Input: dimensioned drawing with shaded views. Units: mm. Origin: part minimum x, y, z. Give positions to 0.01 mm unless a question says otherwise; leave off trailing zeros. Loops run counter-clockwise (first coordinate to the right, second up) from the corner with the lowest first, then second, coordinate; pieces in that order, holes last.
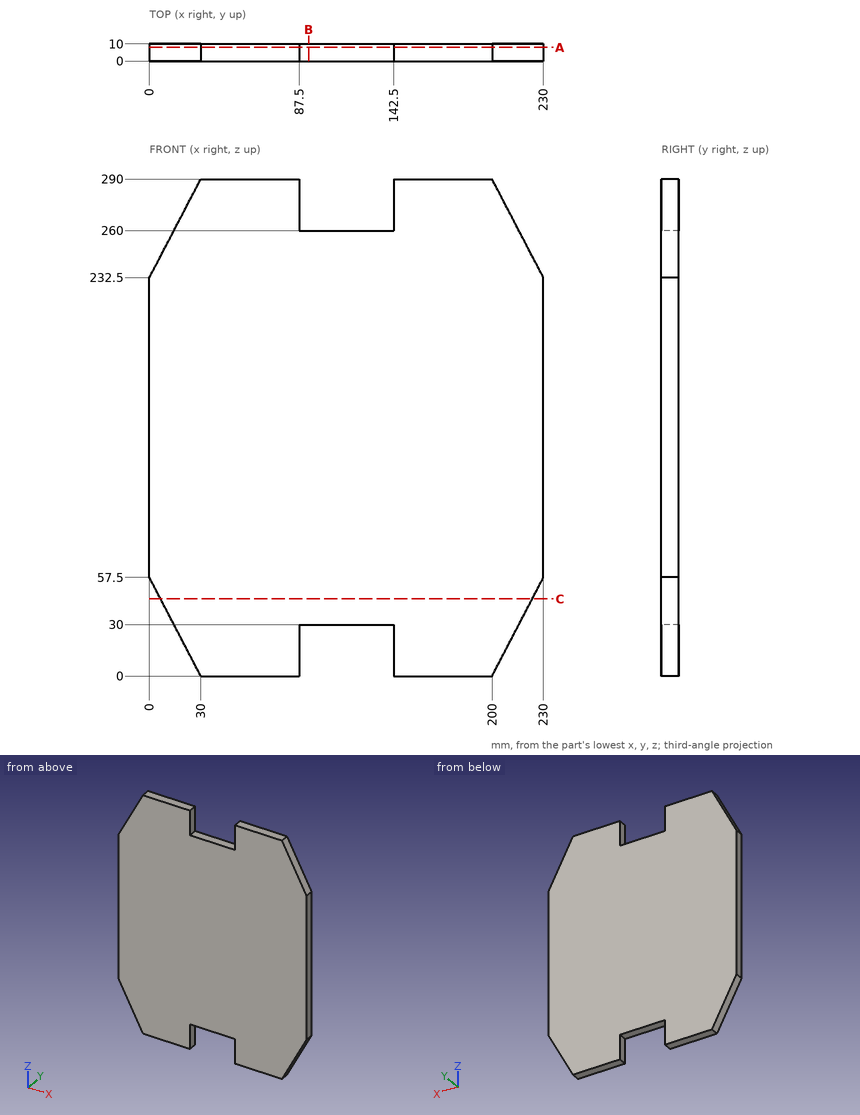
Item 1: Section query A-A on y = 8. Return loops of the section in (x, z).
Values follow:
outline: (0, 57.5) - (30, 0) - (87.5, 0) - (87.5, 30) - (142.5, 30) - (142.5, 0) - (200, 0) - (230, 57.5) - (230, 232.5) - (200, 290) - (142.5, 290) - (142.5, 260) - (87.5, 260) - (87.5, 290) - (30, 290) - (0, 232.5) - close
Item 2: Ray query, probe 1 along X at (y, z) = (4.5, 277); probe 2 along Z at (x, y) = (12, 2.5); probe 3 along Z at (x, y) = (100, 1.5). Return the intervals inside material, ascending.
Values follow:
probe 1: x = 23.22 to 87.5, 142.5 to 206.78
probe 2: z = 34.5 to 255.5
probe 3: z = 30 to 260
Item 3: Pin query (flat end, axial travel): pin 1 (5 mm diameter, centred on x = 104.5, y = 3, fed in from -Z); pin 2 (6 mm diameter, centred on y = 2, z = 239, fed in from -X); pin 3 (4 mm diameter, centred on y = 8, z = 38, fed in from -X). Return the tip coordinate at first contact, or that it passes through.
Values follow:
pin 1: stops at z = 30
pin 2: stops at x = 1.83
pin 3: stops at x = 9.13
Item 4: Section query C-C on z = 45. Return loops of the section in (x, y).
Values follow:
outline: (6.52, 0) - (223.48, 0) - (223.48, 10) - (6.52, 10) - close
Item 5: Section query B-B on x = 93. Return loops of the section in (y, z).
Values follow:
outline: (0, 30) - (10, 30) - (10, 260) - (0, 260) - close
